```python
from build123d import *

# Parameters (mm, degrees)
F0_W     = 139.7
F0_H     = 50.8
F1_DEPTH = 609.6
F2_W     = 46.482
F2_H     = 50.776334
F3_DEPTH = 139.7
F4_W     = 46.482
F4_H     = 50.741273
F5_DEPTH = 139.7


with BuildPart() as f1:
    # F0 (on Top) → F1 (new body)
    with BuildSketch(Plane.XY):
        with Locations((4.855842, 45.481372)):
            Rectangle(F0_W, F0_H)
    extrude(amount=-F1_DEPTH)

    # F2 (on face) → F3 (join)
    with BuildSketch(Plane.XY):
        with Locations((-41.699169, 45.469539)):
            Rectangle(F2_W, F2_H)
    extrude(amount=F3_DEPTH)

    # F4 (on face) → F5 (join)
    with BuildSketch(Plane.XY):
        with Locations((51.438496, 45.510735)):
            Rectangle(F4_W, F4_H)
    extrude(amount=F5_DEPTH)


solid = f1.part
```
Read the model definition and answer for the solid it produces. Units are mm, in the model's axes. A direction names the side the tool comes from. Round coordinates to 2 decimals unless told otherwise and drop trailing zeros. Write each loop counter-clockwise with the first axis right and the second up, starting at its lowest first coordinate (ties: lowest second). Pieces come first, ordered by that corner, then holes. Notation, with made-up numbers: (19, 23) -> (50, 23) arc R31 cw to (50, 56) -> close; hole circle Ø2 at (-11, 47). An arc over 180 degrees is marked (long way). Answer in a Markdown table with one row per item. Add a question column.
1) Find section A-A, the plane z = 28.5. Determine the outline of the cut face in (x, y).
2) Consider line 1 (X direction, y = 42.5, z = 87); line 2 (Z direction, x = 17.5, y = 27); line 3 (Y direction, x = -37, z = 15). Determine where each line is inside the solid, lowest interval first.
3) Which of the six approach directions +Z, -Z, +X, -X, +Y, -Y give full straight-line access (tool end or side, diameter ignored) to faces 1 (the face through (51, 46, 139.7)), 2 (the face through (28.197, 45, 69))?
4) Given P1, Ø15, axis at x = 20.5, y = 43, coming from the +Z side; P2, Ø3, axis at y = 29.5, z = 19.5, coming from the -X side; P3, Ø15, axis at y = 41.5, z = 59, coming from the +X side, each flat-ended and moving along its own axis, determine where each tip first touches the part or whether it passes through.
5) Find section C-C, the plane x = 14.5. Determine the outline of the cut face in (y, z), and give its area (3 significant figures).
6) Determine the mould class of faces 3 (the face through (5, 47, 0)), 4 (the face through (51, 70.881, 69)), 5 (the face through (-64.994, 45, -301)), 6 (the face through (74.679, 45, 69)) for opening direction X: pulls with the +X half, pulls with the -X half, needs draft (parallel to the pull), parting line crosses it, or undercut.
Findings below:
| question | item | result |
|---|---|---|
| 1 | outline | (-64.94, 20.08) -> (-18.46, 20.08) -> (-18.46, 70.86) -> (-64.94, 70.86) -> close; (28.2, 20.14) -> (74.68, 20.14) -> (74.68, 70.88) -> (28.2, 70.88) -> close |
| 2 | line 1 | -64.94 to -18.46, 28.2 to 74.68 |
| 2 | line 2 | -609.6 to 0 |
| 2 | line 3 | 20.08 to 70.86 |
| 3 | face 1 | +Z, +X, -X, +Y, -Y |
| 3 | face 2 | +Z, +Y, -Y |
| 4 | P1 | z = 0 |
| 4 | P2 | x = -64.94 |
| 4 | P3 | x = 74.68 |
| 5 | outline | (20.08, -609.6) -> (70.88, -609.6) -> (70.88, 0) -> (20.08, 0) -> close |
| 5 | area | 31,000 mm² |
| 6 | face 3 | undercut |
| 6 | face 4 | needs draft |
| 6 | face 5 | pulls with the -X half |
| 6 | face 6 | pulls with the +X half |
